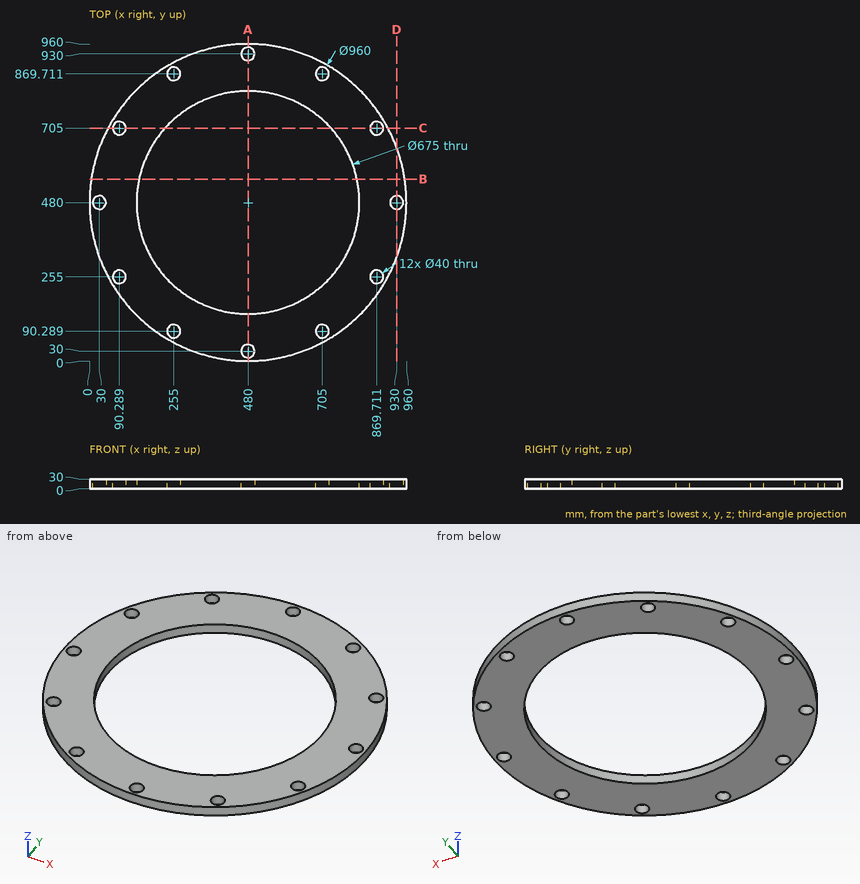
Geometry: see drawing. Coordinates: mm, zero at the bounding-box minimum. Coordinates: 2 decimals unless noted, no trailing zeros. Loops run counter-clockwise (first coordinate to the right, second up) from the corner with the lowest first, then second, coordinate; pieces in that order, holes last. Notation, with made-up numbers: (-21.5, 89.25) - (8.5, 89.25) arc R11 ccw to (8.5, 99.25) - close; hole circle Ø6 at (-16.75, 17.5). An arc over 180 degrees is marked (long way). Return JSON: item names as keys, results as strings.
Q1. Section C-C, the plane y = 705. Return loops of the section in (x, z), plus the area to 3 significant figures.
Results:
{"outline": "(56, 0) - (70.29, 0) - (70.29, 30) - (56, 30) - close; (110.29, 0) - (228.44, 0) - (228.44, 30) - (110.29, 30) - close; (731.56, 0) - (849.71, 0) - (849.71, 30) - (731.56, 30) - close; (889.71, 0) - (904, 0) - (904, 30) - (889.71, 30) - close", "area": "7,950 mm2"}
Q2. Section A-A, the plane x = 480. Return loops of the section in (y, z), plus the area to 3 significant figures.
Results:
{"outline": "(0, 0) - (10, 0) - (10, 30) - (0, 30) - close; (50, 0) - (142.5, 0) - (142.5, 30) - (50, 30) - close; (817.5, 0) - (910, 0) - (910, 30) - (817.5, 30) - close; (950, 0) - (960, 0) - (960, 30) - (950, 30) - close", "area": "6,150 mm2"}
Q3. Section D-D, the plane x = 930. Return loops of the section in (y, z).
Results:
{"outline": "(312.97, 0) - (460, 0) - (460, 30) - (312.97, 30) - close; (500, 0) - (647.03, 0) - (647.03, 30) - (500, 30) - close"}
Q4. Material intervals for line 1 along Y through (x, z) = (480, 13.25); line 2 along Y through (x, z) = (255, 7.5); line 3 along X through (y, z) = (852.5, 14) (1 decimal), sorted ascending.
Results:
{"line 1": "0 to 10, 50 to 142.5, 817.5 to 910, 950 to 960", "line 2": "56 to 70.29, 110.29 to 228.44, 731.56 to 849.71, 889.71 to 904", "line 3": "177.3 to 244.8, 265.2 to 694.8, 715.2 to 782.7"}
Q5. Section B-B, the plane y = 551. Return loops of the section in (x, z), plus the area to 3 significant figures.
Results:
{"outline": "(5.28, 0) - (150.05, 0) - (150.05, 30) - (5.28, 30) - close; (809.95, 0) - (954.72, 0) - (954.72, 30) - (809.95, 30) - close", "area": "8,690 mm2"}
Q6. Contact query for flat-ended pins moving along their axis: P1, Ø4, axis at y = 773, z = 4.5, coming from the +X side; P2, Ø6, axis at x = 406, z = 23, coming from the +Y side; P3, Ø4, axis at y = 305.5, z = 26, coming from the +X side. Output: stop coordinate, or through.
Results:
{"P1": "x = 861.73", "P2": "y = 954.72", "P3": "x = 927.93"}
